Study the drawing (mm; zero at the part's minimum x, y, z) and answer. A direction names the side the tool comes from. Give positions to 0.01 mm unless a question says otherwise; leave off trailing zeros. Write each loop counter-clockwise with the first axis right and the second up, starting at its lowest first coordinate (ties: lowest second). Pieces come first, ordered by that corner, then holes. Notation, with made-up numbers: M -14.5,40.25 L 9.5,40.25 A35 cw 9.5,76.25 Z; hole C 80.25,63.25 d3. An arc over 180 degrees is marked long. Use a Markdown table: item, result. Add a question column.
Item 1: A cutting plane is placed at B-B on y = 5.5. Determine the outline of the cut face in (x, z).
Item 2: A cutting plane is placed at C-C on x = 24. Determine the outline of the cut face in (y, z).
Item 3: For the marked faces 4 and 5, determine the directions among +Z, -Z, +X, -X, +Y, -Y from which every point of the face is accessible in a straight line to the end or side of a thin tool.
Item 4: A cutting plane is placed at D-D on x = 33. Determine the outline of the cut face in (y, z), then the cut area to 3 significant figures.
Item 5: The mould has two halves that part along X. Classify the marked faces 1, 2 and 3: pulls with the +X half, pulls with the -X half, needs draft (parallel to the pull), parting line crosses it, or undercut.
Item 6: Given P1, Ø1.6, axis at x = 38, y = 3, coming from the -Z side; P2, Ø1.8, axis at x = 15.5, y = 4.5, coming from the +Z side, each flat-ended and moving along its own axis, determine where each tip first touches the part or whether it passes through.
Item 7: A cutting plane is placed at A-A on y = 2.25. Determine the outline of the cut face in (x, z) (1 decimal).
Item 8: Consider probe 1 along X at (y, z) = (4, 3); probe 2 along Y at (x, z) = (38, 2.7); probe 3 along X at (y, z) = (3.25, 1.4) (1 decimal). Determine where each line is inside the solid, lowest interval first. Write a range as [from, to].
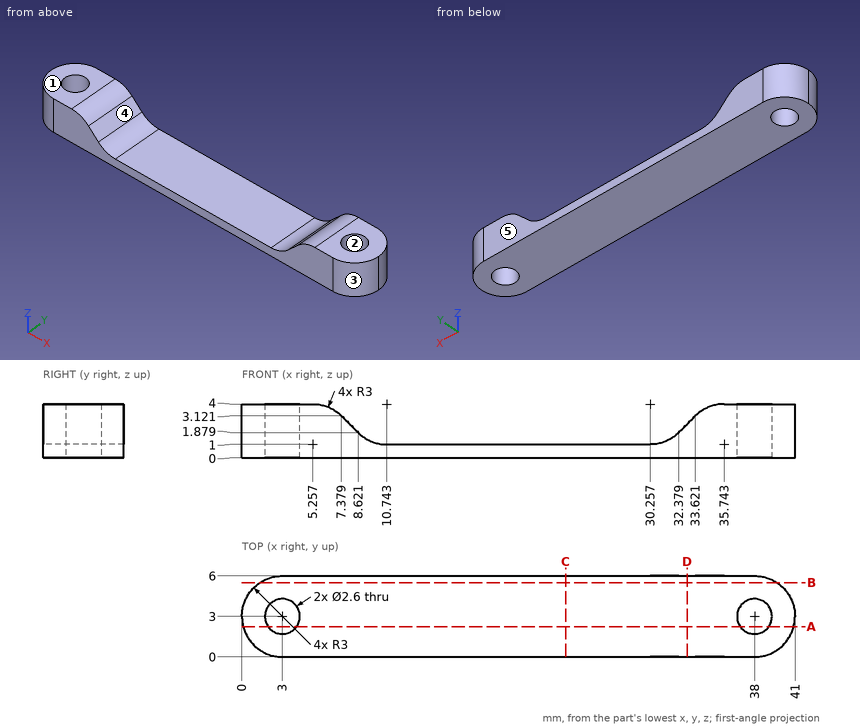
Filled in:
| question | item | result |
|---|---|---|
| 1 | outline | M 1.34,0 L 39.66,0 L 39.66,4 L 35.74,4 A3 ccw 33.62,3.12 L 32.38,1.88 A3 cw 30.26,1 L 10.74,1 A3 cw 8.62,1.88 L 7.38,3.12 A3 ccw 5.26,4 L 1.34,4 Z |
| 2 | outline | M 0,0 L 6,0 L 6,1 L 0,1 Z |
| 3 | face 4 | +Z, +Y, -Y |
| 3 | face 5 | +Z, -Z, +X, -X, +Y |
| 4 | outline | M 0,0 L 6,0 L 6,2.5 L 0,2.5 Z |
| 4 | area | 15.0 mm² |
| 5 | face 1 | needs draft |
| 5 | face 2 | undercut |
| 5 | face 3 | pulls with the +X half |
| 6 | P1 | through |
| 6 | P2 | z = 1 |
| 7 | outline | M 0.1,0 L 1.9,0 L 1.9,4 L 0.1,4 Z; M 4.1,0 L 36.9,0 L 36.9,4 L 35.7,4 A3 ccw 33.6,3.1 L 32.4,1.9 A3 cw 30.3,1 L 10.7,1 A3 cw 8.6,1.9 L 7.4,3.1 A3 ccw 5.3,4 L 4.1,4 Z; M 39.1,0 L 40.9,0 L 40.9,4 L 39.1,4 Z |
| 8 | probe 1 | [0.17, 2.17], [3.83, 7.5], [33.5, 37.17], [38.83, 40.83] |
| 8 | probe 2 | [0, 1.7], [4.3, 6] |
| 8 | probe 3 | [0, 1.7], [4.3, 9.2], [31.8, 36.7], [39.3, 41] |
